Model file for the job. Use its own axes, mm. A direction names the side the tool comes from. Round coordinates to 2 decimals unless told otherwise and drop trailing zeros. Order: outer loops, then holes, each group sorted by start corner. A loop starts at its lowest first (then second) coordinate and runs counter-clockwise, first axis right, second up. Notation, with made-up numbers: (17, 61.5) - (24, 61.5) arc R17 ccw to (24, 80.5) - close; hole circle Ø3 at (-24, 3). An arc over 180 degrees is marked (long way). Write item = value, one per line.
Autodesk Inventor part; units mm, degrees
ref_plane "Work Plane1" through (22.5184, 2.463, -18.3509) normal (0, 0, 1) x (0.9997722, -0.0213418, 0)
ref_plane "YZ Plane" through (0, 0, 0) normal (1, 0, 0) x (0, 1, 0)
ref_plane "XZ Plane" through (0, 0, 0) normal (0, 1, 0) x (-1, 0, 0)
ref_plane "Work Plane1" through (22.5184, 2.463, -18.3509) normal (0, 0, 1) x (0.9997722, -0.0213418, 0)
sketch "ThermoBulbBorder" plane through (22.5184, 2.463, -18.3509) normal (0, 0, 1) x (0.9997722, -0.0213418, 0)
  arc A0 (-447.455, -468.958) -> (162.145, -468.958) centre (-142.655, -774.8145) ccw
  arc A1 (-339.505, -542.1063) -> (98.645, -588.5959) centre (-142.655, -774.8145) ccw
  line L0 (-447.455, -468.958) -> (-339.505, -468.958)
  line L1 (162.145, -468.958) -> (98.645, -468.958)
  line L2 (98.645, -468.958) -> (98.645, -588.5959)
  line L3 (-383.955, -961.033) -> (-484.4967, -1038.6241)
  line L4 (98.645, -961.033) -> (199.1867, -1038.6241)
  arc A2 (-447.455, -468.958) -> (162.145, -468.958) centre (-142.655, -774.8145) ccw
  line L5 (98.645, -468.958) -> (98.645, -316.558) construction
  line L6 (-339.505, -468.958) -> (-339.505, -542.1063)
  line L7 (-383.955, -468.958) -> (-383.955, 914.2855)
  line L8 (-447.455, 914.2855) -> (-447.455, -468.958)
  line L9 (-383.955, -468.958) -> (-383.955, -961.033) construction
  dimension "d0" = 609.6
  dimension "d6" = 63.5
  dimension "d12" = 152.4
  dimension "d53" = 107.95
extrude "Extrusion6" add sketch "ThermoBulbBorder" along normal blind 18.034 contours L0 L6 A1 L3 A0
sketch "Sketch3" plane through (22.5184, 2.463, -0.3169) normal (0, 0, 1) x (0.9997722, -0.0213418, 0)
  arc A0 (-447.455, -468.958) -> (-484.4967, -1038.6241) centre (-142.655, -774.8145) ccw
  line L0 (-484.4967, -1038.6241) -> (-383.955, -961.033)
  arc A1 (-339.505, -542.1063) -> (-383.955, -961.033) centre (-142.655, -774.8145) ccw
  line L1 (-339.505, -468.958) -> (-447.455, -468.958)
  arc A2 (-429.1801, -468.958) -> (-435.8114, -475.308) centre (-142.655, -774.8145) ccw construction
  arc A3 (-436.6135, -493.4561) -> (-464.7905, -1023.4163) centre (-142.655, -774.8145) ccw
  line L2 (-474.4425, -1030.865) -> (-464.7905, -1023.4163)
  arc A4 (-373.4379, -528.461) -> (-409.8948, -981.0515) centre (-142.655, -774.8145) ccw
  line L3 (-142.655, -774.8145) -> (-429.1801, -468.958) construction
  line L4 (-419.5468, -988.5003) -> (-409.8948, -981.0515)
  line L5 (-396.3065, -475.308) -> (-422.6679, -475.308)
  line L6 (-422.6679, -487.5) -> (-396.2592, -487.5)
  arc A5 (-445.4213, -485.0259) -> (-474.4425, -1030.865) centre (-142.655, -774.8145) ccw
  arc A6 (-381.7732, -519.5633) -> (-396.2592, -487.5) centre (-396.2592, -506.804) ccw
  arc A7 (-373.4379, -528.461) -> (-396.3065, -475.308) centre (-396.3065, -506.804) ccw
  arc A8 (-422.6679, -487.5) -> (-436.6135, -493.4561) centre (-422.6679, -506.804) ccw
  arc A9 (-422.6679, -475.308) -> (-445.4213, -485.0259) centre (-422.6679, -506.804) ccw
  arc A10 (-381.7732, -519.5633) -> (-419.5468, -988.5003) centre (-142.655, -774.8145) ccw
  point P0 (-22.4607, -2.943)
  point P1 (-383.955, -468.958)
  point P2 (-430.7947, -487.5)
  dimension "d56" = 12.7
  dimension "d57" = 12.192
  dimension "d61" = 63.5
  dimension "d62" = 6.35
  dimension "d63" = 12.192
  dimension "d64" = 19.304
  dimension "d65" = 31.496
  dimension "d66" = 19.304
  dimension "d67" = 31.496
  dimension "d68" = 57.15
  dimension "d69" = 12.192
extrude "Extrusion7" cut sketch "Sketch3" against normal blind 12.7 contours A5 A9 L5 A7 A4 L0 A10 A6 L6 A8 A3
equation "\"d6\" = d5"
equation "\"d57\" = bRopeChannel"
equation "\"d63\" = bRopeChannel"
equation "\"d69\" = bRopeChannel"
equation "\"bRopeChannel\" = 12.192"
equation "\"d8\" = bRopeChannel"
equation "\"d9\" = bRopeChannel"
equation "\"d38\" = bRopeChannel"
equation "\"d60\" = bRopeChannel"
properties part number "HOT Thermo bulb outline L" material "Rubber, Butyl"
1) Cut at A-A (z = -4.75). Write the cut outline in (x, y).
Conclusion:
outline = (-484.03, -1025.58) - (-473.82, -1018.04) arc R419.1 cw to (-433.15, -472.95) arc R31.5 cw to (-410.2, -463.72) - (-383.84, -464.28) arc R31.5 cw to (-362.11, -517.91) arc R337.57 ccw to (-408.22, -969.62) - (-381.86, -950.16) arc R304.8 cw to (-328.48, -532.27) - (-326.92, -459.14) - (-434.84, -456.84) arc R431.8 ccw to start; (-464.01, -1010.8) - (-418.03, -976.86) arc R349.76 cw to (-370.26, -508.83) arc R19.3 ccw to (-384.05, -476.47) - (-410.46, -475.91) arc R19.3 ccw to (-424.53, -481.56) arc R406.91 ccw to start
2) Flat gauge pins, fed straight in: pin 1 Ø1 at (x, z) = (-368.5, -4) entering from +Y; pin 2 Ø10 at (y, z) = (-708.5, -12) entering from +X; pin 3 Ø4 at (x, z) = (-530, -14) entering from +Y. Where does each tip first touch, or does it go through?
Conclusion:
pin_1 = -458.24
pin_2 = -434.29
pin_3 = -586.68
3) Wall check: line 1 along X through (y, z) = (-810, -10.75); line 2 along X through (y, z) = (-773, -12.5); line 3 along Y through (x, z) = (-394, -1). Give the ranges that are in metal, low to high.
Conclusion:
line_1 = -566.5 to -553.74, -541.49 to -484, -471.72 to -438.69
line_2 = -568.42 to -555.72, -543.53 to -486.38, -474.18 to -441.42
line_3 = -959.12 to -932.44, -605.82 to -550.69, -532.28 to -476.26, -464.06 to -457.71
4) Mould opens along Y. For faces 1 (the face through (-472.09, -731.39, -6.58)), 2 (the face through (-459, -719, -0.317)), 3 (the face through (-432.23, -987.34, -9.46)) say: +Y half, -Y half, draft (parallel to the pull), parting line (faces both ways), or undercut.
Conclusion:
face_1 = undercut
face_2 = draft
face_3 = -Y half
5) Cut at B-B (x = -505.5). Write the cut outline in (y, z).
Conclusion:
outline = (-993.62, -18.35) - (-544.65, -18.35) - (-544.65, -0.32) - (-570.17, -0.32) - (-570.17, -13.02) - (-597.33, -13.02) - (-597.33, -0.32) - (-940.93, -0.32) - (-940.93, -13.02) - (-968.1, -13.02) - (-968.1, -0.32) - (-993.62, -0.32) - close
6) 3-axis set-ups, long thin cutter, end or side, ignore diameter. For faces 4 (the face through (-484.205, -730.023, -6.578)), 5 (the face through (-439.38, -733.74, -9.46)): which of +Z, -Z, +X, -X, +Y, -Y reach the whole face in a straight line?
Conclusion:
face_4 = +Z
face_5 = +Z, -Z, +X
7) Cut at D-D (x = -452). Write the cut outline in (y, z), and give its area (3 significant figures).
Conclusion:
outline = (-1001.94, -18.35) - (-474.17, -18.35) - (-474.17, -0.32) - (-493.1, -0.32) - (-493.1, -13.02) - (-511.99, -13.02) - (-511.99, -0.32) - (-617.87, -0.32) - (-617.87, -13.02) - (-648.72, -13.02) - (-648.72, -0.32) - (-889.54, -0.32) - (-889.54, -13.02) - (-920.39, -13.02) - (-920.39, -0.32) - (-1001.94, -0.32) - close
area = 8,490 mm^2
8) Cut at C-C (y = -490.5). Write the cut outline in (x, z).
Conclusion:
outline = (-466.51, -18.35) - (-327.59, -18.35) - (-327.59, -0.32) - (-353.46, -0.32) - (-353.46, -13.02) - (-365.9, -13.02) - (-365.9, -0.32) - (-433.19, -0.32) - (-433.19, -13.02) - (-449.71, -13.02) - (-449.71, -0.32) - (-466.51, -0.32) - close
